The model under review builds one solid part; all positions refer to its coordinate system, in mm. A direction names the side the tool comes from. Coordinates: 2 decimals unless noted, no trailing zeros. Loops run counter-clockwise (first coordinate to the right, second up) from the corner with the lowest first, then second, coordinate; pieces in that order, holes last. Notation, with made-up numbers: (71, 47) - (115, 47) arc R32 ccw to (115, 82) - close; hole circle Ø11 at (-16, 2). An arc over 180 degrees is marked (long way). Answer in a Markdown table with one row per item. Add a question column.
(1) Mouldability with a two-part tool opening along Z and no side actions: class faces 1 (the flat face through (6, 0, 0)), 2 (the flat face through (0, -6, 2)), 3 (the cylindrical face through (-10.316, -7.91, 26.241)) as +Z half, -Z half, draft (parallel to the pull), parting line (faces both ways), or undercut.
(2) We need section A-A on x = 0. Write out the cut boundary in (y, z).
(3) For line 1 along Y through (x, z) = (0, 1.1); line 2 along Z through (x, y) = (-2.5, 23); line 3 along Z through (x, y) = (11.5, 7.5), list the stretches that pass through material, from the lowest coordinate up.
(4) Machinability: for faces 4 (the cylindrical face through (-29.97, 1.32, 4.44)), 5 (the cylindrical face through (25.865, -10.724, 4.958)), 6 (the cylindrical face through (-14.985, 0.66, 26.762)), which of the approach directions +Z, -Z, +X, -X, +Y, -Y give a long, thin tool a straight path to every point of the face, cutting with its end or side? Answer none if there is none.
(5) We need section C-C on z = 22. Write out the cut boundary in (x, y).
(6) For P1, Ø12, axis at x = 15, z = 29.5, coming from the -Y side; P2, Ø1, axis at y = -8, z = 29, coming from the +X side; P3, Ø1.5, axis at x = -7.5, z = 28.5, coming from the +Y side, all flat-tipped, find the tip position at first contact; note any pin that passes through.
from build123d import *

# Parameters (mm, degrees)
CROQUIS1_R              = 30
SALIENTE_EXTRUIR1_DEPTH = 10
CROQUIS2_R              = 15
SALIENTE_EXTRUIR2_DEPTH = 35
VACIADO1_T              = -2
REDONDEO1_R             = 1
REDONDEO2_R             = 1
CORTAR_EXTRUIR1_REACH   = 62.407
CROQUIS3_R              = 5


with BuildPart() as part:
    # Croquis1 → Saliente-Extruir1 (new body)
    with BuildSketch(Plane.XY):
        Circle(CROQUIS1_R)
    extrude(amount=SALIENTE_EXTRUIR1_DEPTH)

    # Croquis2 → Saliente-Extruir2 (add)
    with BuildSketch(Plane.XY.offset(10)):
        Circle(CROQUIS2_R)
    extrude(amount=SALIENTE_EXTRUIR2_DEPTH)

    # Vaciado1
    vaciado1_openings = [part.faces().sort_by_distance(p)[0] for p in [
        (0, 0, 45),
    ]]
    offset(amount=VACIADO1_T, openings=vaciado1_openings, kind=Kind.INTERSECTION)

    # Redondeo1
    redondeo1_edges = [part.edges().sort_by_distance(p)[0] for p in [
        (-30, 0, 10),
    ]]
    fillet(redondeo1_edges, radius=REDONDEO1_R)

    # Redondeo2
    redondeo2_edges = [part.edges().sort_by_distance(p)[0] for p in [
        (-15, 0, 45),
    ]]
    fillet(redondeo2_edges, radius=REDONDEO2_R)

    # Croquis3 → Cortar-Extruir1 (cut, up to next)
    with BuildSketch(Plane.XY.offset(2), mode=Mode.PRIVATE) as cortar_extruir1_sk1:
        Circle(CROQUIS3_R)
    cortar_extruir1_tool1 = extrude(cortar_extruir1_sk1.sketch, amount=-CORTAR_EXTRUIR1_REACH, mode=Mode.PRIVATE) & part.part
    add(cortar_extruir1_tool1.solids().sort_by_distance((0, 0, 2))[0], mode=Mode.SUBTRACT)


solid = part.part
Outcome:
| question | item | result |
|---|---|---|
| 1 | face 1 | -Z half |
| 1 | face 2 | undercut |
| 1 | face 3 | draft |
| 2 | outline | (-30, 0) - (-5, 0) - (-5, 2) - (-28, 2) - (-28, 8) - (-13, 8) - (-13, 45) - (-14, 45) arc R1 ccw to (-15, 44) - (-15, 10) - (-29, 10) arc R1 ccw to (-30, 9) - close; (5, 0) - (30, 0) - (30, 9) arc R1 ccw to (29, 10) - (15, 10) - (15, 44) arc R1 ccw to (14, 45) - (13, 45) - (13, 8) - (28, 8) - (28, 2) - (5, 2) - close |
| 3 | line 1 | -30 to -5, 5 to 30 |
| 3 | line 2 | 0 to 2, 8 to 10 |
| 3 | line 3 | 0 to 2, 8 to 45 |
| 4 | face 4 | +Z, -Z |
| 4 | face 5 | none |
| 4 | face 6 | +Z |
| 5 | outline | circle Ø30 at (0, 0); hole circle Ø26 at (0, 0) |
| 6 | P1 | y = -12 |
| 6 | P2 | x = 12.99 |
| 6 | P3 | y = 13.4 |
